```python
from build123d import *

# Parameters (mm, degrees)
SKETCH1_W            = 63.384201813
SKETCH1_H            = 99.23964582
BOSS_EXTRUDE1_DEPTH  = 4
M5_CLEARANCE_HOLE1_D = 5.3
FILLET1_R            = 10
M5_CLEARANCE_HOLE2_D = 6
M3_CLEARANCE_HOLE1_D = 3.2


with BuildPart() as part:
    # Sketch1 → Boss-Extrude1 (new body)
    with BuildSketch(Plane.XY):
        with Locations((-76.771477461, -317.489186132)):
            Rectangle(SKETCH1_W, SKETCH1_H)
        with BuildLine():
            Line((-63.453357461, -301.557900971), (-89.297127128, -301.557900971))
            ThreePointArc((-89.297127128, -301.557900971), (-90.004233909, -301.265007752), (-90.297127128, -300.557900971))
            Line((-90.297127128, -300.557900971), (-90.297127128, -289.479666407))
            ThreePointArc((-90.297127128, -289.479666407), (-90.004233909, -288.772559625), (-89.297127128, -288.479666407))
            Line((-89.297127128, -288.479666407), (-63.453357461, -288.479666407))
            ThreePointArc((-63.453357461, -288.479666407), (-62.74625068, -288.772559625), (-62.453357461, -289.479666407))
            Line((-62.453357461, -289.479666407), (-62.453357461, -300.557900971))
            ThreePointArc((-62.453357461, -300.557900971), (-62.74625068, -301.265007752), (-63.453357461, -301.557900971))
        make_face(mode=Mode.SUBTRACT)
    extrude(amount=BOSS_EXTRUDE1_DEPTH)

    # M5 Clearance Hole1 (through all)
    with Locations(Plane.XY.offset(4)):
        with Locations((-54.16270611, -321.915681156), (-54.16270611, -293.415681156)):
            Hole(M5_CLEARANCE_HOLE1_D / 2)

    # Fillet1
    fillet1_edges = [part.edges().sort_by_distance(p)[0] for p in [
        (-108.463578367, -267.869363222, 2),
        (-45.079376554, -267.869363222, 2),
        (-45.079376554, -367.109009042, 2),
        (-108.463578367, -367.109009042, 2),
    ]]
    fillet(fillet1_edges, radius=FILLET1_R)

    # M5 Clearance Hole2 (through all)
    with Locations(Plane(origin=(0, 0, 0), x_dir=(-1, 0, 0), z_dir=(0, 0, -1))):
        with Locations((54.617319332, -359.802896905)):
            Hole(M5_CLEARANCE_HOLE2_D / 2)

    # M3 Clearance Hole1 (through all)
    with Locations(Plane.XY.offset(4)):
        with Locations((-98.463578367, -357.109009042), (-98.463578367, -277.869363222)):
            Hole(M3_CLEARANCE_HOLE1_D / 2)


solid = part.part
```
Verification items for the finished model (mm, model axes). A direction names the side the tool comes from. Give positions to 0.01 mm unless a question says otherwise; leave off trailing zeros. Loops run counter-clockwise (first coordinate to the right, second up) from the corner with the lowest first, then second, coordinate; pieces in that order, holes last.
1. Go/stop test with flat-tipped pins: pin 1 Ø6 at (x, y) = (-54.16, -321.92) entering from -Z; pin 2 Ø5 at (x, y) = (-76, -292) entering from -Z. Record where each tip stops, or that it passes through.
2. Mould release check, pull along X, two halves, no side actions. Record for faces 3 (the flat face through (-77, -288.48, 2)), 4 (the flat face through (-45.079, -318, 2)), 5 (the cylindrical face through (-99.32, -276.52, 1.97)), 6 (the flat face through (-77, -367.109, 2)): released by +X, released by -X, zero draft, split by the parting line, or undercut.
3. Section check B-B, the plane z = 3.2. Enter the section's corners in (x, y).
4. Thickness scan on line 1 (Y direction, x = -78, z = 2.8); line 2 (X direction, y = -292, z = 2.8); line 3 (X direction, y = -358.5, z = 2.75). Record the ranges inside material, lowest first.
5. Section check C-C, the plane y = -323. Enter the section's corners in (x, z), then the cut area to 3 significant figures.
6. Set-up check for faces 1 (the flat face through (-77, -317, 4)), 2 (the flat face through (-90.297, -295, 2)): record each of +Z, -Z, +X, -X, +Y, -Y from which the full face is reachable in a straight line by a thin tool's end or side.
7. Section check A-A, the plane x = -87.5. Enter the section's corners in (y, z).
Geometry says:
1. pin 1: stops at z = 0
1. pin 2: passes through
2. face 3: undercut
2. face 4: released by +X
2. face 5: undercut
2. face 6: zero draft
3. outline: (-108.46, -357.11) arc R10 ccw to (-98.46, -367.11) - (-55.08, -367.11) arc R10 ccw to (-45.08, -357.11) - (-45.08, -277.87) arc R10 ccw to (-55.08, -267.87) - (-98.46, -267.87) arc R10 ccw to (-108.46, -277.87) - close; hole circle Ø3.2 at (-98.46, -357.11); hole circle Ø3.2 at (-98.46, -277.87); hole (-90.3, -300.56) arc R1 ccw to (-89.3, -301.56) - (-63.45, -301.56) arc R1 ccw to (-62.45, -300.56) - (-62.45, -289.48) arc R1 ccw to (-63.45, -288.48) - (-89.3, -288.48) arc R1 ccw to (-90.3, -289.48) - close; hole circle Ø6 at (-54.62, -359.8); hole circle Ø5.3 at (-54.16, -321.92); hole circle Ø5.3 at (-54.16, -293.42)
4. line 1: y = -367.11 to -301.56, -288.48 to -267.87
4. line 2: x = -108.46 to -90.3, -62.45 to -56.4, -51.92 to -45.08
4. line 3: x = -108.37 to -99.25, -97.67 to -57.32, -51.92 to -45.18
5. outline: (-108.46, 0) - (-56.58, 0) - (-56.58, 4) - (-108.46, 4) - close; (-51.74, 0) - (-45.08, 0) - (-45.08, 4) - (-51.74, 4) - close
5. area: 234 mm2
6. face 1: +Z, +X, -X, +Y, -Y
6. face 2: +Z, -Z
7. outline: (-367.11, 0) - (-301.56, 0) - (-301.56, 4) - (-367.11, 4) - close; (-288.48, 0) - (-267.87, 0) - (-267.87, 4) - (-288.48, 4) - close
